The figure shows three views and two pictorial views of one solid part (mm, origin at its lowest corner). Answer the questions. Round coordinates to 2 decimals unless told otherwise and drop trailing zeros. Order: outer loops, then holes, each group sorted by start corner. A loop starts at its lowest first (then second) coordinate and runs counter-clockwise, first axis right, second up. Notation, with made-up numbers: (-39, -32.75) -> (7, -32.75) arc R25 ccw to (7, -11.75) -> close; hole circle Ø6 at (9.5, 45.25). An arc over 180 degrees is marked (long way). Return JSON: item names as keys, results as strings. Group by question number.
(1) The part is cut by section A-A (z = 2.55). Determine the outline of the cut face in (x, y).
(2) Consider line 1 (Y direction, x = 34, z = 2.6); line 2 (X direction, y = 36, z = 2.2) (1 decimal); line 3 (X direction, y = 26, z = 3.6) (1 decimal). Determine where each line is inside the solid, lowest interval first. Write a range as [from, to].
(3) The part is cut by section B-B (x = 34). Determine the outline of the cut face in (y, z).
(4) The part is cut by section C-C (y = 30). Determine the outline of the cut face in (x, z), plus the area to 3 significant figures.
(5) The part is cut by section D-D (y = 13.5). Determine the outline of the cut face in (x, z).
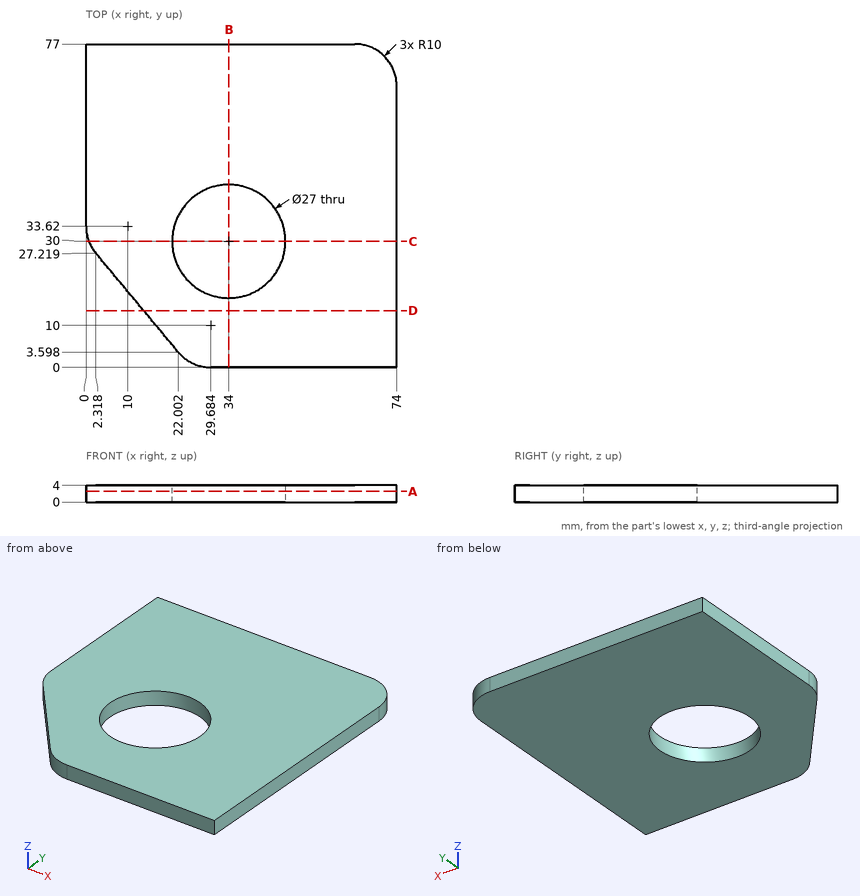
Answer below:
{
 "1": {"outline": "(0, 33.62) arc R10 ccw to (2.32, 27.22) -> (22, 3.6) arc R10 ccw to (29.68, 0) -> (74, 0) -> (74, 67) arc R10 ccw to (64, 77) -> (0, 77) -> close; hole circle Ø27 at (34, 30)"},
 "2": {"line 1": "y = [0, 16.5], [43.5, 77]", "line 2": "x = [0, 21.9], [46.1, 74]", "line 3": "x = [3.3, 21.1], [46.9, 74]"},
 "3": {"outline": "(0, 0) -> (16.5, 0) -> (16.5, 4) -> (0, 4) -> close; (43.5, 0) -> (77, 0) -> (77, 4) -> (43.5, 4) -> close"},
 "4": {"outline": "(0.68, 0) -> (20.5, 0) -> (20.5, 4) -> (0.68, 4) -> close; (47.5, 0) -> (74, 0) -> (74, 4) -> (47.5, 4) -> close", "area": "185 mm²"},
 "5": {"outline": "(13.75, 0) -> (74, 0) -> (74, 4) -> (13.75, 4) -> close"}
}
